For this review, take the finished solid that the model builds, in its own axes (mm). A direction names the side the tool comes from. Coordinates: 2 decimals unless noted, no trailing zeros. Loops run counter-clockwise (first coordinate to the right, second up) from the corner with the lowest first, then second, coordinate; pieces in that order, holes last. Notation, with made-up numbers: (55.5, 81.25) - (102.5, 81.25) arc R28 cw to (102.5, 114.25) - close; hole circle Ø7 at (33, -7). An arc over 180 degrees is marked (long way). Answer as a JSON object with one key per item and string values. Group by question number.
Item 1: To check wall thickness, follow line 1 (X direction, y = 22.5, z = -7); line 2 (Y direction, x = 18.5, z = -22); line 3 (Y direction, x = -40.5, z = 133). State the ranges of each line that lie inside material, in increasing order.
Item 2: We need section C-C (x = 73). Give the boundary of the cut face in (y, z), then the cut area to 3 significant figures.
Item 3: Mouldability with a two-part tool opening along X and no side actions: class faces 1 (the flat face through (-41, 3, 2)), 2 (the cylindrical face through (108.804, 1.711, 2.1)), 3 (the flat face through (-30, 14, 2)), 4 (the flat face through (107, 14, 2)) as released by +X, released by -X, zero draft, split by the parting line, or undercut.
Item 4: Tool access review of faces 5 (the flat face through (26.2, 25.5, -150)), 6 (the cylindrical face through (-28.804, 1.711, 2.1)), 7 (the flat face through (122, 3, 2)): name each direction out of +Z, -Z, +X, -X, +Y, -Y from which nothing blocks a thin tool from reaching the whole face with its end or side.
Item 5: Clearance check with flat-ended pins moving along their axes: pin 1 (13 mm diameter, centred on y = 12, z = -27, fed in from +X); pin 2 (5 mm diameter, centred on x = 119.5, z = -31.5, fed in from +Y); pin 3 (13 mm diameter, centred on y = 14, z = -64, fed in from -X). State where each tip first meets the part, or that it passes through.
Item 6: We need section A-A (y = 19). Give the boundary of the cut face in (x, z), then the cut area to 3 significant figures.
Item 7: We need section B-B (z = -95). Give the boundary of the cut face in (x, y), then the cut area to 3 significant figures.
from build123d import *

# Parameters (mm, degrees)
F0_W        = 140
F0_H        = 25
F1_DEPTH    = 150
F2_T        = 3
F2_T3_DEPTH = 306
F3_R        = 3
F4_R        = 6


# Not quite as in the source:
# - a shell that OpenCascade refuses in one call is made with other operations: the cavity is built on its own and cut out


with BuildPart() as f1:
    # F0 (on Top) → F1 (new body, symmetric)
    with BuildSketch(Plane.XY):
        with Locations((40, 15.5)):
            Rectangle(F0_W, F0_H)
        Polygon((110, 3), (-30, 3), (-50, 3), (-50, 0), (130, 0), (130, 3), align=None)
    extrude(amount=F1_DEPTH, both=True)

    # F2: shell of thickness 3, made by hand


with BuildPart() as f2_core1:
    # F2_t2: copy of F1
    add(f1.part)

    # the walls: a layer under each face that stays
    f2_faces = [f2_core1.faces().sort_by_distance(p)[0] for p in [
        (-30, 15.5, 0),
        (40, 28, 0),
        (110, 15.5, 0),
        (120, 3, 0),
        (130, 1.5, 0),
        (-50, 1.5, 0),
        (-40, 3, 0),
    ]]
    thicken(f2_faces, amount=-F2_T, mode=Mode.SUBTRACT)

    # F2_s4 → F2_t3 (cut)
    with BuildSketch(Plane.XY.offset(-153)):
        Polygon((-30.03, 3.03), (-27, 3), (-27, 0), (-30, 0), align=None)
        Polygon((110.03, 3.03), (107, 3), (107, 0), (110, 0), align=None)
    extrude(amount=F2_T3_DEPTH, mode=Mode.SUBTRACT)


with BuildPart() as f1_1:
    add(f1.part)

    # what is left inside the walls is the cavity
    f2_cavity = [f2_core1.part.solids().sort_by_distance(p)[0] for p in [
        (40, 0.03, -50),
    ]]
    add(f2_cavity, mode=Mode.SUBTRACT)

    # F3
    f3_edges = [f1_1.edges().sort_by_distance(p)[0] for p in [
        (-30, 3, 0),
        (110, 3, 0),
        (-27, 25, 0),
        (107, 25, 0),
    ]]
    fillet(f3_edges, radius=F3_R)

    # F4
    f4_edges = [f1_1.edges().sort_by_distance(p)[0] for p in [
        (-27, 0, 0),
        (107, 0, 0),
        (-30, 28, 0),
        (110, 28, 0),
    ]]
    fillet(f4_edges, radius=F4_R)


solid = f1_1.part
Check sheet entries:
{
 "1": {"line 1": "x = -29.98 to -26.96, 106.96 to 109.98", "line 2": "y = 25 to 28", "line 3": "y = 0 to 3"},
 "2": {"outline": "(25, -150) - (28, -150) - (28, 150) - (25, 150) - close", "area": "900 mm2"},
 "3": {"face 1": "zero draft", "face 2": "undercut", "face 3": "released by -X", "face 4": "undercut"},
 "4": {"face 5": "-Z, +X, -X, +Y, -Y", "face 6": "+Z, -Z, -Y", "face 7": "+Z, -Z, +X, +Y"},
 "5": {"pin 1": "stops at x = 110.04", "pin 2": "stops at y = 3", "pin 3": "stops at x = -30"},
 "6": {"outline": "(-30, -150) - (-27, -150) - (-27, 150) - (-30, 150) - close; (107, -150) - (110, -150) - (110, 150) - (107, 150) - close", "area": "1,800 mm2"},
 "7": {"outline": "(-50, 0) - (-33, 0) arc R6 ccw to (-27, 6) - (-27, 22) arc R3 cw to (-24, 25) - (104, 25) arc R3 cw to (107, 22) - (107, 6) arc R6 ccw to (113, 0) - (130, 0) - (130, 3) - (113, 3) arc R3 cw to (110, 6) - (110, 22) arc R6 ccw to (104, 28) - (-24, 28) arc R6 ccw to (-30, 22) - (-30, 6) arc R3 cw to (-33, 3) - (-50, 3) - close", "area": "667 mm2"}
}
